The figure shows three views and two pictorial views of one solid part (mm, origin at its lowest corner). Answer the questions. A direction names the side the tool comes from. Coordinates: 2 decimals unless noted, no trailing zeros. Loops run counter-clockwise (first coordinate to the right, second up) from the corner with the lowest first, then second, coordinate; pieces in that order, holes last. Notation, with made-up numbers: M 5,-19.75 L 57,-19.75 A11 ccw 57,-1.75 Z; hole C 75,2.25 d9. An arc over 180 degrees is marked long. One line per item, written item: value. Start each with the question number.
1. The part is cut by section D-D (x = 24). Write down the section's boundary in (y, z) (1 decimal).
2. For the marked faces 1 and 2, determine the directions among +Z, -Z, +X, -X, +Y, -Y from which every point of the face is accessible in a straight line to the end or side of a thin tool.
3. The part is cut by section A-A (y = 19.05). Write down the section's boundary in (x, z) (1 decimal), then the cut area to 3 significant figures.
4. Consider probe 1 along Y at (x, z) = (19, 60); probe 2 along Z at (x, y) = (10, 8.5); probe 3 along Y at (x, z) = (19.5, 22.5) (1 decimal). Determine where each line is inside the solid, lowest interval first.
5. Flat-ended cylindrical pins translate along their axes: pin 1 (1.5 mm diameter, centred on x = 28, y = 9, fed in from +Z); pin 2 (5 mm diameter, centred on x = 23, z = 14.5, fed in from +Y) (1 decimal); pin 3 (8 mm diameter, centred on x = 30, z = 47, fed in from +Y); pin 4 (12 mm diameter, centred on x = 6, y = 9, fed in from -Z). Find the tip coordinate at first contact, or state that the pin passes through.
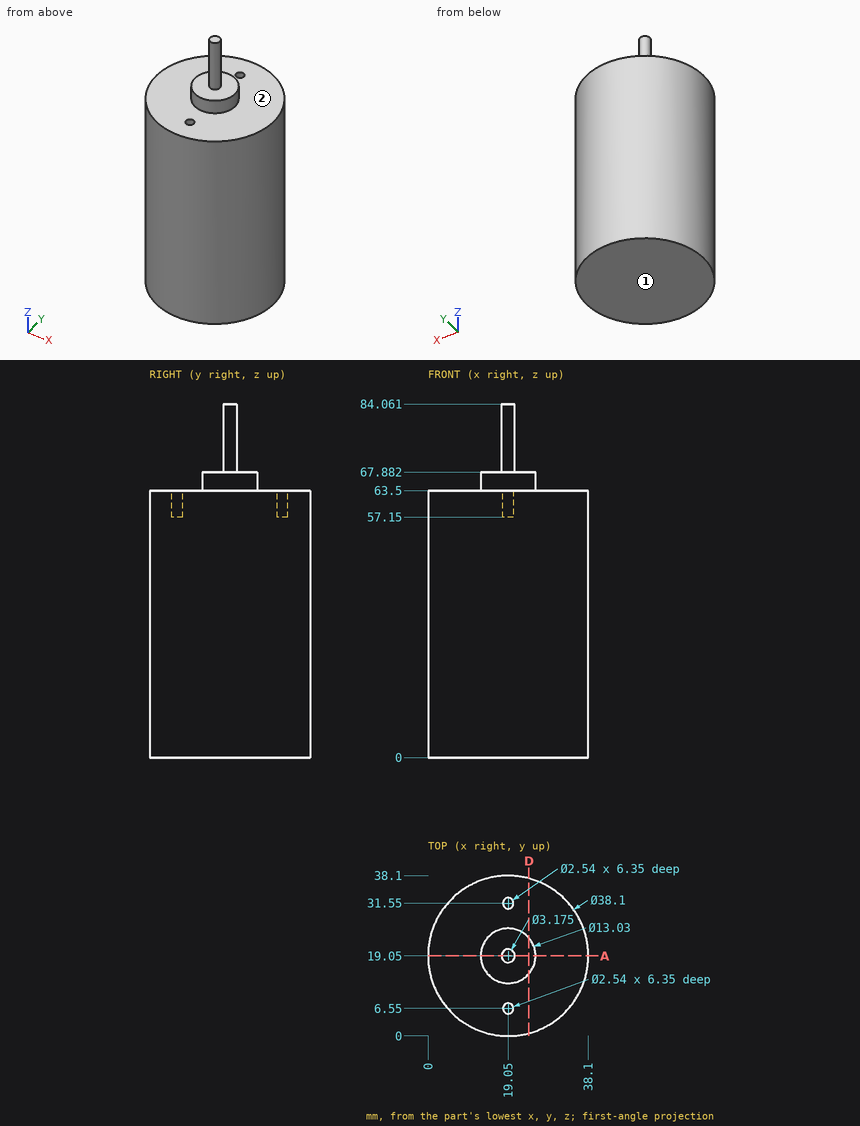
Answer block:
1. outline: M 0.7,0 L 37.4,0 L 37.4,63.5 L 23.3,63.5 L 23.3,67.9 L 14.8,67.9 L 14.8,63.5 L 0.7,63.5 Z
2. face 1: -Z, +X, -X, +Y, -Y
2. face 2: +Z
3. outline: M 0,0 L 38.1,0 L 38.1,63.5 L 25.6,63.5 L 25.6,67.9 L 20.6,67.9 L 20.6,84.1 L 17.5,84.1 L 17.5,67.9 L 12.5,67.9 L 12.5,63.5 L 0,63.5 Z
3. area: 2,530 mm2
4. probe 1: y = 0 to 5.28, 7.82 to 30.28, 32.82 to 38.1
4. probe 2: z = 0 to 63.5
4. probe 3: y = 0 to 38.1
5. pin 1: stops at z = 63.5
5. pin 2: stops at y = 38
5. pin 3: stops at y = 36.79
5. pin 4: stops at z = 0
